```python
from build123d import *

# Parameters (mm, degrees)
CONG_1_R                                        = 1
ESQUISSE2_R                                     = 1.2
ENL_V_MAT_EXTRU_1_DEPTH                         = 23.649503412
CHAMBRAGE_POUR_VIS_T_TE_CYLINDRIQUE_D           = 2.4
CHAMBRAGE_POUR_VIS_T_TE_CYLINDRIQUE_CBORE_D     = 6.5
CHAMBRAGE_POUR_VIS_T_TE_CYLINDRIQUE_CBORE_DEPTH = 1.5
ESQUISSE3_R                                     = 1.5
ENL_V_MAT_EXTRU_2_DEPTH                         = 23.649503478


with BuildPart() as part:
    # Esquisse1 → Révolution1 (revolve)
    with BuildSketch(Plane.XY, mode=Mode.PRIVATE) as r_volution1_sk:
        with BuildLine():
            Line((3.1, 15), (3.1, 1))
            Line((3.1, 1), (4, 1))
            Line((4, 1), (4, 0))
            Line((4, 0), (12, 0))
            Line((12, 0), (12, 3))
            Line((12, 3), (8.013575778, 5.260181833))
            ThreePointArc((8.013575778, 5.260181833), (7.271872626, 5.993234994), (7, 7))
            Line((7, 7), (7, 15))
            Line((7, 15), (3.1, 15))
        make_face()
    revolve(r_volution1_sk.sketch.rotate(Axis((0, 0, 0), (0, 1, 0)), 90), axis=Axis((0, 0, 0), (0, 1, 0)))

    # Congé1
    cong_1_edges = [part.edges().sort_by_distance(p)[0] for p in [
        (0, 15, 7),
        (0, 3, 12),
    ]]
    fillet(cong_1_edges, radius=CONG_1_R)

    # Esquisse2 → Enlèv. mat.-Extru.1 (cut, through all)
    with BuildSketch(Plane.XZ):
        with Locations(Location((-10, 0, 0), (0, 0, 270))):
            Circle(ESQUISSE2_R)
        with Locations(Location((10, 0, 0), (0, 0, 270))):
            Circle(ESQUISSE2_R)
    extrude(amount=-ENL_V_MAT_EXTRU_1_DEPTH, mode=Mode.SUBTRACT)

    # Chambrage pour vis à tête cylindrique à 6 pans creux (ou vis CHC) M31 (through all)
    with Locations(Plane(origin=(0, 11, 7), x_dir=(1, 0, 0), z_dir=(0, 0, 1))):
        with Locations((0, 0)):
            CounterBoreHole(CHAMBRAGE_POUR_VIS_T_TE_CYLINDRIQUE_D / 2, CHAMBRAGE_POUR_VIS_T_TE_CYLINDRIQUE_CBORE_D / 2, CHAMBRAGE_POUR_VIS_T_TE_CYLINDRIQUE_CBORE_DEPTH)

    # Esquisse3 → Enlèv. mat.-Extru.2 (cut, through all)
    with BuildSketch(Plane.XY):
        with Locations(Location((0, 11, 0), (0, 0, 180))):
            Circle(ESQUISSE3_R)
    extrude(amount=ENL_V_MAT_EXTRU_2_DEPTH, mode=Mode.SUBTRACT)


solid = part.part
```
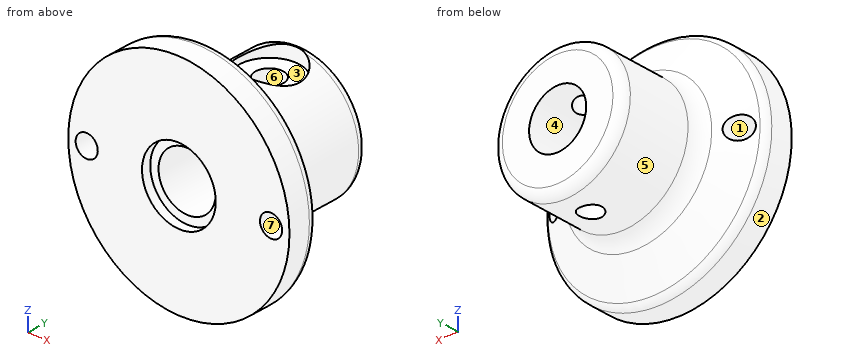
Part model, mm, in its own coordinate system. Face numbers are marked on the shaded views. A direction names the side the tool comes from. Coordinates: 2 decimals unless noted, no trailing zeros. Order: outer loops, then holes, each group sorted by start corner. A loop starts at its lowest first (then second) coordinate and runs counter-clockwise, first axis right, second up. Notation, with made-up numbers: (-1, -6) -> (12, -6) arc R18 ccw to (12, 22) -> close; hole circle Ø1 at (21, -23). An arc over 180 degrees is marked (long way). Put each result on its own line as item: value. Start each with the question number.
(1) Band-saw the part on A-A (y = 11). Give the cut face in (x, z), then the cut area to 3 significant figures.
(2) Band-saw the part on B-B (x = 0). Count the separate pieces of the cut face and the enclosed holes in it, then the cut area to 3 significant figures.
(3) Band-saw the part on D-D (y = 1.5). Give the cut face in (x, z).
(4) Pin check, flat tips, straight feed: pin 1 Ø5 at (x, y) = (0, 11) entering from +Z; pin 2 Ø1.8 at (x, y) = (0, 11) entering from +Z; pin 3 Ø1 at (x, y) = (-4.5, 9) entering from +Z; pin 4 Ø3 at (x, y) = (-7, 5.5) entering from +Z. Stop position of each tip, or through.
(5) Probe line 1 along X through (y, z) = (1.4, 0); line 2 along X through (y, z) = (0.55, 0); line 3 along X through (y, z) = (10.75, 0). List the from-to ranges inside material, lowest first. Write a range as [from, to].
(6) Which spindle directions (+Z, -Z, +X, -X, +Y, -Y) get a long thin tool onto all of the face, cutting with end or side? Do the marked faces 5, 6 and 7. Say none if no direction does.
(7) Mould opens along Z. For the marked faces 1, 2, 3 and 4 say: pulls with the +Z half, pulls with the -Z half, needs draft (parallel to the pull), parting line crosses it, or undercut.
Determined:
1. outline: (-3.25, 5.5) -> (-3.25, 6.2) arc R7 ccw to (-1.2, -6.9) -> (-1.2, -2.86) arc R3.1 cw to (-1.5, 2.71) -> (-1.5, 5.5) -> close; (1.2, -6.9) arc R7 ccw to (3.25, 6.2) -> (3.25, 5.5) -> (1.5, 5.5) -> (1.5, 2.71) arc R3.1 cw to (1.2, -2.86) -> close
1. area: 98.6 mm²
2. separate pieces: 4
2. enclosed holes: 0
2. area: 133 mm²
3. outline: circle Ø24 at (0, 0); hole circle Ø2.4 at (-10, 0); hole circle Ø6.2 at (0, 0); hole circle Ø2.4 at (10, 0)
4. pin 1: stops at z = 5.5
4. pin 2: passes through
4. pin 3: stops at z = 5.74
4. pin 4: stops at z = 7.71
5. line 1: x = [-12, -11.2], [-8.8, -3.1], [3.1, 8.8], [11.2, 12]
5. line 2: x = [-12, -11.2], [-8.8, -4], [4, 8.8], [11.2, 12]
5. line 3: x = [-7, -3.1], [3.1, 7]
6. face 5: +Y
6. face 6: +Z
6. face 7: +Y, -Y
7. face 1: undercut
7. face 2: parting line crosses it
7. face 3: pulls with the +Z half
7. face 4: undercut
